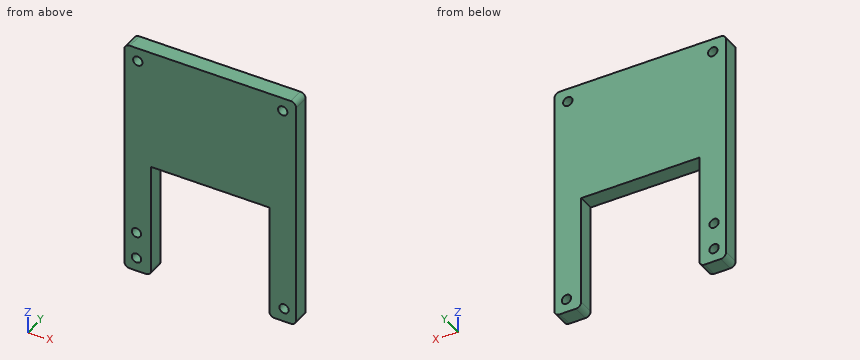
from build123d import *

# Parameters (mm, degrees)
F0_W     = 64
F0_H     = 88
F1_DEPTH = 6
F2_R     = 1.75
F3_DEPTH = 25
F4_R     = 2


# Not quite as in the source:
# - a feature names something its author has since deleted; it is built from what else it names


with BuildPart() as f1:
    # F0 (on Front) → F1 (new body)
    with BuildSketch(Plane.XZ):
        Rectangle(F0_W, F0_H)
    extrude(amount=F1_DEPTH)

    # F2 (on face) → F3 (cut)
    with BuildSketch(Plane.XZ.offset(6)):
        Polygon((22, -1), (0, -1), (-22, -1), (-22, -44), (22, -44), align=None)
        with Locations((27.5, -39)):
            Circle(F2_R)
        with Locations((-27.5, -29)):
            Circle(F2_R)
        with Locations((-27.5, -39)):
            Circle(F2_R)
        with Locations((-27, 39)):
            Circle(F2_R)
        with Locations((27, 39)):
            Circle(F2_R)
    extrude(amount=-F3_DEPTH, mode=Mode.SUBTRACT)

    # F4
    f4_edges = [f1.edges().sort_by_distance(p)[0] for p in [
        (-32, -3, 44),
        (32, -3, 44),
        (-32, -3, -44),
        (32, -3, -44),
        (-22, -3, -44),
        (22, -3, -44),
    ]]
    fillet(f4_edges, radius=F4_R)


solid = f1.part
The listing builds one solid part. Answer for the finished solid, in the listing's coordinates (mm). Coordinates: 2 decimals unless noted, no trailing zeros. Loops run counter-clockwise (first coordinate to the right, second up) from the corner with the lowest first, then second, coordinate; pieces in that order, holes last.
1) Find section C-C on y = -3.05. Write down the section's boundary in (x, z), then the cut area to 3 significant figures.
2) Find section B-B on z = -29. Write down the section's boundary in (x, y), then the cut area to 3 significant figures.
3) Find the intervals of material crossed by L1, parallel to Z at x = -27.5, y = -4.2; L2, parallel to X at y = -1.2, z = -32; L3, parallel to Z at x = -29, y = -5.35, in increasing order.
4) Find section D-D on z = -6. Write down the section's boundary in (x, y), then the cut area to 3 significant figures.
5) Find section A-A on z = -39. Write down the section's boundary in (x, y), then the cut area to 3 significant figures.
6) Flat-ended cylindrical pins translate along their axes: pin 1 Ø3 at (x, z) = (-27, 39) entering from +Y; pin 2 Ø3 at (x, z) = (11.5, 2.5) entering from +Y; pin 3 Ø1.8 at (x, y) = (-1.5, -3.5) entering from -Z. Find the tip coordinate at first contact, or state that the pin passes through.
Values:
1. outline: (-32, -42) arc R2 ccw to (-30, -44) - (-24, -44) arc R2 ccw to (-22, -42) - (-22, -1) - (22, -1) - (22, -42) arc R2 ccw to (24, -44) - (30, -44) arc R2 ccw to (32, -42) - (32, 42) arc R2 ccw to (30, 44) - (-30, 44) arc R2 ccw to (-32, 42) - close; hole circle Ø3.5 at (-27.5, -39); hole circle Ø3.5 at (-27.5, -29); hole circle Ø3.5 at (-27, 39); hole circle Ø3.5 at (27, 39); hole circle Ø3.5 at (27.5, -39)
1. area: 3,690 mm2
2. outline: (-32, -6) - (-29.25, -6) - (-29.25, 0) - (-32, 0) - close; (-25.75, -6) - (-22, -6) - (-22, 0) - (-25.75, 0) - close; (22, -6) - (32, -6) - (32, 0) - (22, 0) - close
2. area: 99.0 mm2
3. L1: z = -44 to -40.75, -37.25 to -30.75, -27.25 to 37.32, 40.68 to 44
3. L2: x = -32 to -22, 22 to 32
3. L3: z = -44 to -39.9, -38.1 to -29.9, -28.1 to 44
4. outline: (-32, -6) - (-22, -6) - (-22, 0) - (-32, 0) - close; (22, -6) - (32, -6) - (32, 0) - (22, 0) - close
4. area: 120 mm2
5. outline: (-32, -6) - (-29.25, -6) - (-29.25, 0) - (-32, 0) - close; (-25.75, -6) - (-22, -6) - (-22, 0) - (-25.75, 0) - close; (22, -6) - (25.75, -6) - (25.75, 0) - (22, 0) - close; (29.25, -6) - (32, -6) - (32, 0) - (29.25, 0) - close
5. area: 78.0 mm2
6. pin 1: passes through
6. pin 2: stops at y = 0
6. pin 3: stops at z = -1
